Design review of the part built by this model. Coordinates are the model's own, in mm. Give positions to 0.01 mm unless a question says otherwise; leave off trailing zeros. Order: outer loops, then holes, each group sorted by start corner. A loop starts at its lowest first (then second) coordinate and runs counter-clockwise, first axis right, second up. Notation, with made-up numbers: (44.25, -24.5) -> (98.25, -24.5) arc R23 ccw to (98.25, -5.5) -> close; hole circle Ø11 at (85, 86.25). An arc over 180 degrees is marked (long way). One line per item, written item: value.
from build123d import *

# Parameters (mm, degrees)
BOSS_EXTRUDE1_DEPTH = 1
SKETCH2_W           = 10
SKETCH2_H           = 5
CUT_EXTRUDE1_DEPTH  = 1


with BuildPart() as part:
    # Sketch1 → Boss-Extrude1 (new body)
    with BuildSketch(Plane(origin=(0, 0, 0), x_dir=(1, 0, 0), z_dir=(0, 1, 0))):
        with BuildLine():
            Line((-22.5, -12.500000317), (-22.5, 12.500000317))
            Line((-22.5, 12.500000317), (22.5, 12.500000317))
            Line((22.5, 12.500000317), (22.5, -12.499999683))
            add(Edge.make_bspline(
                [(-22.5, -12.500000317), (-22.439792168, -12.471062497), (-21.720318389, -12.126671398), (-20.033278548, -11.358209685), (-16.487166751, -9.929593391), (-11.649258831, -8.428412522), (-5.831090838, -7.344665325), (-7.7e-08, -6.981224033), (5.831090693, -7.344665161), (11.649258717, -8.428412194), (16.487166679, -9.929592927), (20.033278516, -11.358209122), (21.720318379, -12.126670787), (22.439792167, -12.471061866), (22.5, -12.499999683)],
                knots=[0.029712498, 0.029712498, 0.029712498, 0.029712498, 0.033515652, 0.075187399, 0.135874913, 0.257249942, 0.378624971, 0.5, 0.621375029, 0.742750058, 0.864125087, 0.924812601, 0.966484348, 0.970287502, 0.970287502, 0.970287502, 0.970287502], degree=3))
        make_face()
    extrude(amount=BOSS_EXTRUDE1_DEPTH)

    # Sketch2 → Cut-Extrude1 (cut)
    with BuildSketch(Plane(origin=(0, 1, 0), x_dir=(1, 0, 0), z_dir=(0, 1, 0))):
        with Locations((-10.5, -1.999999683)):
            Rectangle(SKETCH2_W, SKETCH2_H)
    extrude(amount=-CUT_EXTRUDE1_DEPTH, mode=Mode.SUBTRACT)


solid = part.part
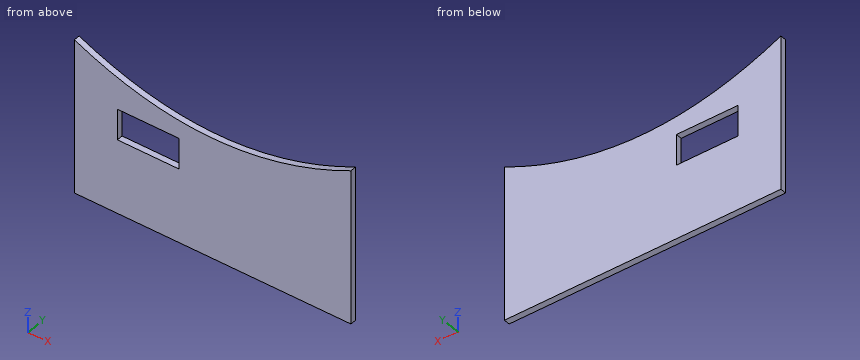
Item 1: Add section A-A on z = 2. Give the boundary of the cut face in (x, y), plus the area to 3 significant figures.
Returned:
outline: (-22.5, 0) -> (-15.5, 0) -> (-15.5, 1) -> (-22.5, 1) -> close; (-5.5, 0) -> (22.5, 0) -> (22.5, 1) -> (-5.5, 1) -> close
area: 35.0 mm²
Item 2: Clearance check with flat-ended pins moving along their axes: P1, Ø0.5, axis at x = -10, y = 0.5, coming from the +Z side; P2, Ø3, axis at x = 17.5, z = 4.5, coming from the -Y side. State where each tip first meets the part, or that it passes through.
Returned:
P1: z = 8.22
P2: y = 0
Item 3: To check wall thickness, follow line 1 along X through (y, z) = (0.5, 2.75); line 2 along Z through (x, y) = (15.5, 0.6); line 3 along Z through (x, y) = (6, 0.3). State the ranges of each line that lie inside material, in increasing order. Write a range as from..to.
Returned:
line 1: -22.5..-15.5, -5.5..22.5
line 2: -12.5..9.66
line 3: -12.5..7.49
